from build123d import *

# Parameters (mm, degrees)
F0_W      = 160
F0_H      = 160
F1_DEPTH  = 50
F2_T      = -2.5
F4_DEPTH  = 25
F6_DEPTH  = 25
F8_DEPTH  = 25
F10_DEPTH = 25
F11_W     = 120
F11_H     = 120
F12_DEPTH = 25
F13_R     = 5
F14_R     = 1


with BuildPart() as f1:
    # F0 (on Front) → F1 (new body)
    with BuildSketch(Plane.XZ):
        Rectangle(F0_W, F0_H)
    extrude(amount=F1_DEPTH)

    # F2
    f2_openings = [f1.faces().sort_by_distance(p)[0] for p in [
        (0, 0, 0),
    ]]
    offset(amount=F2_T, openings=f2_openings)

    # F3 (on face) → F4 (cut)
    with BuildSketch(Plane(origin=(0, 0, -80), x_dir=(1, 0, 0), z_dir=(0, 0, -1))):
        with BuildLine():
            Line((-40, 0), (40, 0))
            ThreePointArc((40, 0), (0, 40), (-40, 0))
        make_face()
    extrude(amount=-F4_DEPTH, mode=Mode.SUBTRACT)

    # F5 (on face) → F6 (cut)
    with BuildSketch(Plane(origin=(-80, 0, 0), x_dir=(0, -1, 0), z_dir=(-1, 0, 0))):
        with BuildLine():
            Line((0, 39.9988864115), (0, -39.9988864115))
            ThreePointArc((0, -39.9988864115), (39.7015274931, 0), (0, 39.9988864115))
        make_face()
    extrude(amount=-F6_DEPTH, mode=Mode.SUBTRACT)

    # F7 (on face) → F8 (cut)
    with BuildSketch(Plane.XY.offset(80)):
        with BuildLine():
            Line((40, 0), (-40, 0))
            ThreePointArc((-40, 0), (0, -40), (40, 0))
        make_face()
    extrude(amount=-F8_DEPTH, mode=Mode.SUBTRACT)

    # F9 (on face) → F10 (cut)
    with BuildSketch(Plane.YZ.offset(80)):
        with BuildLine():
            Line((0, -39.999914752), (0, 39.999914752))
            ThreePointArc((0, 39.999914752), (-40.0825822808, 0), (0, -39.999914752))
        make_face()
    extrude(amount=-F10_DEPTH, mode=Mode.SUBTRACT)

    # F11 (on face) → F12 (cut)
    with BuildSketch(Plane.XZ.offset(50)):
        Rectangle(F11_W, F11_H)
    extrude(amount=-F12_DEPTH, mode=Mode.SUBTRACT)

    # F13
    f13_edges = [f1.edges().sort_by_distance(p)[0] for p in [
        (80, -25, 80),
        (0, -50, 80),
        (80, -50, 0),
        (80, -25, -80),
        (0, -50, -80),
        (-80, -25, -80),
        (-80, -50, 0),
        (-80, -25, 80),
    ]]
    fillet(f13_edges, radius=F13_R)

    # F14
    f14_edges = [f1.edges().sort_by_distance(p)[0] for p in [
        (0, -40, -77.5),
        (0, -40, -80),
        (77.5, -40.082582, 0),
        (80, -40.082582, 0),
        (0, -40, 77.5),
        (0, -40, 80),
        (-77.5, -39.701527, 0),
        (-80, -39.701527, 0),
    ]]
    fillet(f14_edges, radius=F14_R)


solid = f1.part
Design review of the part built by this model. Coordinates are the model's own, in mm. A direction names the side the tool comes from. Give positions to 0.01 mm unless a question says otherwise; leave off trailing zeros. Order: outer loops, then holes, each group sorted by start corner. A loop starts at its lowest first (then second) coordinate and runs counter-clockwise, first axis right, second up.
1. Add section D-D, the plane x = -66. State the section outline as (y, z) points.
Solution:
outline: (-50, -75) arc R5 ccw to (-45, -80) - (0, -80) - (0, -77.5) - (-47.5, -77.5) - (-47.5, 77.5) - (0, 77.5) - (0, 80) - (-45, 80) arc R5 ccw to (-50, 75) - close
2. Add section B-B, the plane x = 0. State the section outline as (y, z) points, then the cut area to 3 significant figures.
Solution:
outline: (-50, -75) arc R5 ccw to (-45, -80) - (-41, -80) arc R1 ccw to (-40, -79) - (-40, -78.5) arc R1 ccw to (-41, -77.5) - (-47.5, -77.5) - (-47.5, -60) - (-50, -60) - close; (-50, 60) - (-47.5, 60) - (-47.5, 77.5) - (-41, 77.5) arc R1 ccw to (-40, 78.5) - (-40, 79) arc R1 ccw to (-41, 80) - (-45, 80) arc R5 ccw to (-50, 75) - close
area: 126 mm2
3. Add section A-A, the plane z = 0. State the section outline as (x, y) points, then the cut area to 3 significant figures.
Solution:
outline: (-80, -45) arc R5 ccw to (-75, -50) - (-60, -50) - (-60, -47.5) - (-77.5, -47.5) - (-77.5, -40.7) arc R1 ccw to (-78.5, -39.7) - (-79, -39.7) arc R1 ccw to (-80, -40.7) - close; (60, -50) - (75, -50) arc R5 ccw to (80, -45) - (80, -41.08) arc R1 ccw to (79, -40.08) - (78.5, -40.08) arc R1 ccw to (77.5, -41.08) - (77.5, -47.5) - (60, -47.5) - close
area: 126 mm2
4. Add section C-C, the plane z = -65. State the section outline as (x, y) points.
Solution:
outline: (-80, -45) arc R5 ccw to (-75, -50) - (75, -50) arc R5 ccw to (80, -45) - (80, 0) - (77.5, 0) - (77.5, -47.5) - (-77.5, -47.5) - (-77.5, 0) - (-80, 0) - close
5. Tool access review of faces 4 (the flat face through (-1, -42, -80)), 5 (the flat face through (-70, -47.5, 1)): name each direction out of +Z, -Z, +X, -X, +Y, -Y from which nothing blocks a thin tool from reaching the whole face with its end or side.
Solution:
face 4: -Z, +X, -X, +Y, -Y
face 5: +Y
6. Mouldability with a two-part tool opening along X and no side actions: class faces 1 (the flat face through (80, -42, -1)), 2 (the flat face through (-1, -45, 77.5)), 3 (the flat face through (-68, -50, 1)) as +X half, -X half, draft (parallel to the pull), parting line (faces both ways), or undercut.
Solution:
face 1: +X half
face 2: undercut
face 3: draft
7. For pin 1 Ø0.8 at (y, z) = (-48.5, 9) entering from -X; pin 2 Ø1.2 at (x, y) = (-4.5, -48.5) entering from +Z; pin 3 Ø10 at (x, y) = (34, -6.5) entering from -Z; pin 4 Ø2 at (y, z) = (-48.5, -30) entering from +X, all flat-tipped, find the tip position at first contact; note any pin that passes through.
Solution:
pin 1: stops at x = -78.92
pin 2: stops at z = 79.07
pin 3: passes through
pin 4: stops at x = 79.33
8. To check wall thickness, follow L1, parallel to X at y = -31, z = -52.5; L2, parallel to Y at x = 68, z = -68.5. State the ranges of each line that lie inside material, in increasing order.
Solution:
L1: x = -80 to -77.5, 77.5 to 80
L2: y = -50 to -47.5
